Can you work these out from the model? Positions are in its coordinate system, mm. A direction names the side the tool comes from. Round coordinates to 2 decimals unless told otherwise and drop trailing zeros. Write each loop counter-clockwise with the first axis right and the second up, starting at its lowest first coordinate (ties: lowest second). Pieces come first, ordered by that corner, then holes. Notation, with made-up numbers: (16.25, 57) -> (67.25, 57) arc R5 cw to (67.25, 65) -> close; hole circle Ø8 at (-29, 62.5). An arc over 180 degrees is marked (long way). Use CSV: the item, a comma, the result in double quotes.
```python
from build123d import *

# Parameters (mm, degrees)
EXTRUDE_1_DEPTH     = 10
CUT_EXTRUDE_1_DEPTH = 78.662529175
SKETCH_3_W          = 48.53
SKETCH_3_H          = 1.8
SKETCH_3_W_2        = 69.1
SKETCH_3_H_2        = 2.4
CUT_EXTRUDE_2_DEPTH = 80.403046846
CUT_EXTRUDE_3_DEPTH = 80.403046846
CHAMFER_1_SIZE      = 0.6


with BuildPart() as part:
    # 草图1 → 凸台-拉伸1 (new body)
    with BuildSketch(Plane(origin=(0, 0, 0), x_dir=(1, 0, 0), z_dir=(0, 1, 0))):
        Polygon((-14.635948, 19.40625), (-14.635948, 10.60625), (-12.135948, 10.60625), (-12.135948, 9.40625), (71.996502, 9.40625), (71.996502, 10.40625), (76.364052, 10.40625), (76.364052, 19.40625), align=None)
    extrude(amount=EXTRUDE_1_DEPTH)

    # 草图2 → 切除-拉伸1 (cut, through all)
    with BuildSketch(Plane.XY.offset(-9.40625)):
        Polygon((-14.635948, 9), (67.526731656, 9), (76.526731656, 0), (-14.635948, 0), align=None)
        Polygon((78.332625034, 0.315426966), (67.430737892, 11.217314108), (78.393598105, 11.217314108), align=None)
    extrude(amount=-CUT_EXTRUDE_1_DEPTH, mode=Mode.SUBTRACT)

    # 草图3 → 切除-拉伸2 (cut, through all)
    with BuildSketch(Plane(origin=(0, 10, 0), x_dir=(1, 0, 0), z_dir=(0, 1, 0))):
        with Locations((9.629052, 16.84625)):
            Rectangle(SKETCH_3_W, SKETCH_3_H)
        with Locations((27.674052, 10.60625)):
            Rectangle(SKETCH_3_W_2, SKETCH_3_H_2)
    extrude(amount=-CUT_EXTRUDE_2_DEPTH, mode=Mode.SUBTRACT)

    # 草图4 → 切除-拉伸3 (cut, through all)
    with BuildSketch(Plane(origin=(0, 10, 0), x_dir=(1, 0, 0), z_dir=(0, 1, 0))):
        with BuildLine():
            Line((12.170037326, 15.94625), (18.770037326, 15.94625))
            ThreePointArc((18.770037326, 15.94625), (19.759986819, 15.536199494), (20.170037326, 14.54625))
            Line((20.170037326, 14.54625), (20.170037326, 14.048022825))
            ThreePointArc((20.170037326, 14.048022825), (19.759986819, 13.058073332), (18.770037326, 12.648022825))
            Line((18.770037326, 12.648022825), (12.170037326, 12.648022825))
            ThreePointArc((12.170037326, 12.648022825), (11.180087832, 13.058073332), (10.770037326, 14.048022825))
            Line((10.770037326, 14.048022825), (10.770037326, 14.54625))
            ThreePointArc((10.770037326, 14.54625), (11.180087832, 15.536199494), (12.170037326, 15.94625))
        make_face()
    extrude(amount=-CUT_EXTRUDE_3_DEPTH, mode=Mode.SUBTRACT)

    # 倒角1
    chamfer_1_edges = [part.edges().sort_by_distance(p)[0] for p in [
        (-14.635948, 9.5, -15.94625),
        (-14.635948, 9.5, -17.74625),
    ]]
    chamfer(chamfer_1_edges, length=CHAMFER_1_SIZE)


solid = part.part
```
Q1. Will these pins go through, and if not, where does the flat tip stop? P1, Ø1.1, axis at x = 5, y = 9.5, coming from the +Z side; P2, Ø1, axis at x = 18.5, z = -17, coming from the -Y side; P3, Ø1.1, axis at y = 9.5, z = -11, coming from the +X side; P4, Ø1.1, axis at x = -13, y = 9.5, coming from the +Z side.
Resolved:
P1,"stops at z = -11.81"
P2,"passes through"
P3,"stops at x = 69.7"
P4,"stops at z = -10.61"
Q2. Suppose I cut it at A-A (x = 3.5). Write out the boundary of the cut face in (y, z).
Resolved:
outline,"(9, -19.41) -> (10, -19.41) -> (10, -17.75) -> (9, -17.75) -> close; (9, -15.95) -> (10, -15.95) -> (10, -11.81) -> (9, -11.81) -> close"
Q3. Suppose I cut it at D-D (x = 64). Write out the boundary of the cut face in (y, z).
Resolved:
outline,"(9, -19.41) -> (10, -19.41) -> (10, -9.41) -> (9, -9.41) -> close"
Q4. If we mould it in two halves opening along Z, with no side actions, what happens to faces 1 (the face through (26, 9, -14)), 2 (the face through (19.8, 9.5, -13.1)), 3 (the face through (11.19, 9.51, -13.05)), 4 (the face through (68, 9, -9.406))? For each: released by +Z, released by -Z, zero draft, split by the parting line, or undercut.
Resolved:
face 1,"zero draft"
face 2,"undercut"
face 3,"undercut"
face 4,"released by +Z"
Q5. Please list where these lines run through material, in increasing order: probe 1 along Y at (x, z) = (24.5, -12); probe 2 along Z at (x, y) = (5, 9.5); probe 3 along Z at (x, y) = (52, 9.5).
Resolved:
probe 1,"y = 9 to 10"
probe 2,"z = -19.41 to -17.75, -15.95 to -11.81"
probe 3,"z = -19.41 to -11.81"
Q6. Suppose I cut it at B-B (z = -16.75). Write out the boundary of the cut face in (x, y).
Resolved:
outline,"(33.89, 9) -> (67.53, 9) -> (76.36, 0.16) -> (76.36, 2.28) -> (68.65, 10) -> (33.89, 10) -> close"
Q7. On a 3-axis mill with a long thin cutter (end or side, diameter ignored), from which of +Z, -Z, +X, -X, +Y, -Y can I reach the whole of each face in a straight line? I mean faces 5 (the face through (74, 3, -10.406)), 6 (the face through (34.4, 9.4, -19.406)), 7 (the face through (11.169, 9.507, -15.525)). Say none if no direction works.
Resolved:
face 5,"+Z, +X, +Y, -Y"
face 6,"-Z, +X, -X, +Y, -Y"
face 7,"+Y, -Y"
Q8. Suppose I cut it at C-C (x = 14.5). Write out the boundary of the cut face in (y, z), and give its area (3 significant figures).
Resolved:
outline,"(9, -19.41) -> (10, -19.41) -> (10, -17.75) -> (9, -17.75) -> close; (9, -12.65) -> (10, -12.65) -> (10, -11.81) -> (9, -11.81) -> close"
area,"2.50 mm^2"
